Design review of the part built by this model. Coordinates are the model's own, in mm. Coordinates: 2 decimals unless noted, no trailing zeros. Write each loop counter-clockwise with the first axis right and the second up, starting at its lowest first coordinate (ties: lowest second). Pieces come first, ordered by that corner, then holes. Notation, with made-up numbers: (8.25, 8.5) -> (17.25, 8.5) arc R13 ccw to (17.25, 12.5) -> close; hole circle Ø2 at (-6.75, -32). An arc over 180 degrees is marked (long way). Write item = value, one per line. Start each with the question number.
```python
from build123d import *

# Parameters (mm, degrees)
F0_W     = 76.2
F0_H     = 25.4
F1_DEPTH = 9.525
F2_D     = 3.7973


with BuildPart() as f1:
    # F0 (on Top) → F1 (new body)
    with BuildSketch(Plane.XY):
        Rectangle(F0_W, F0_H)
    extrude(amount=-F1_DEPTH)

    # F2 (through all)
    with Locations(Plane.XY):
        with Locations((-25.4, 0), (25.4, 0), (0, 0)):
            Hole(F2_D / 2)


solid = f1.part
```
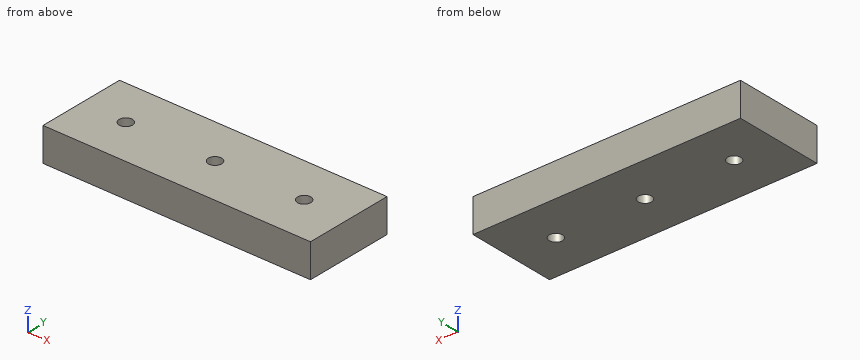
(1) Take a section at C-C, the plane y = 0. State the section outline as (x, z) points (3 decimals), then the cut area to 3 significant figures.
(2) Take a section at A-A, the plane x = 25.4. State the section outline as (y, z) points (3 decimals), then the cut area to 3 significant figures.
(3) For pin 1 Ø3.5 at (x, y) = (25.4, 0) entering from -Z, flat-tipped, find the tip position at first contact; note if it passes through.
(4) Take a section at B-B, the plane z = -7.75. State the section outline as (x, y) points, then the cut area to 3 significant figures.
(5) For line 1 (Y direction, x = -25.4, z = -4.5); line 2 (Y direction, x = 24, z = -2), list the stretches that pass through material, from the lowest coordinate up.
Report:
q1.outline = (-38.1, -9.525) -> (-27.299, -9.525) -> (-27.299, 0) -> (-38.1, 0) -> close; (-23.501, -9.525) -> (-1.899, -9.525) -> (-1.899, 0) -> (-23.501, 0) -> close; (1.899, -9.525) -> (23.501, -9.525) -> (23.501, 0) -> (1.899, 0) -> close; (27.299, -9.525) -> (38.1, -9.525) -> (38.1, 0) -> (27.299, 0) -> close
q1.area = 617 mm2
q2.outline = (-12.7, -9.525) -> (-1.899, -9.525) -> (-1.899, 0) -> (-12.7, 0) -> close; (1.899, -9.525) -> (12.7, -9.525) -> (12.7, 0) -> (1.899, 0) -> close
q2.area = 206 mm2
q3.pin_1 = through
q4.outline = (-38.1, -12.7) -> (38.1, -12.7) -> (38.1, 12.7) -> (-38.1, 12.7) -> close; hole circle Ø3.8 at (-25.4, 0); hole circle Ø3.8 at (0, 0); hole circle Ø3.8 at (25.4, 0)
q4.area = 1,900 mm2
q5.line_1 = -12.7 to -1.9, 1.9 to 12.7
q5.line_2 = -12.7 to -1.28, 1.28 to 12.7
